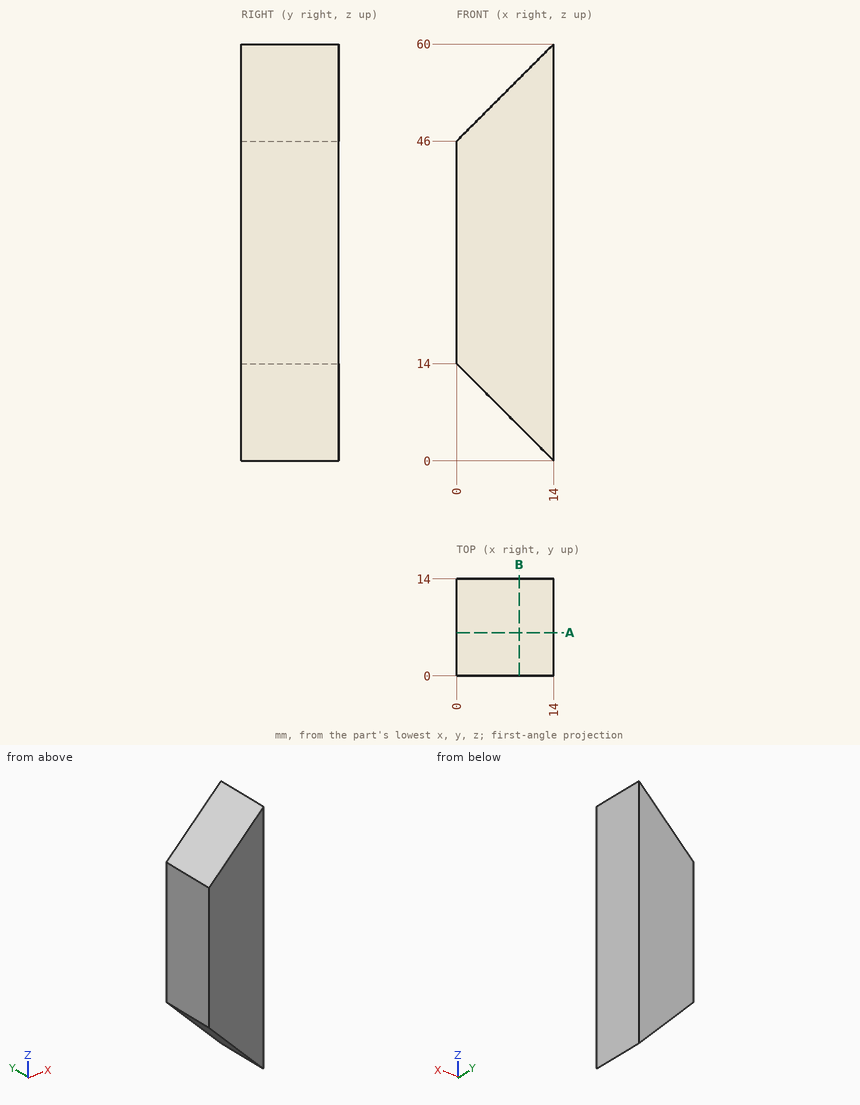
Check sheet for the drawn part. Datum: minimum x, y, z corner. Units: mm. Round coordinates to 2 decimals unless told otherwise and drop trailing zeros. Write each loop counter-clockwise with the first axis right and the second up, starting at its lowest first coordinate (ties: lowest second). Pieces come first, ordered by that corner, then holes. Notation, with made-up numbers: (64, 89.25) - (104, 89.25) arc R22 cw to (104, 111.25) - close; hole circle Ø10 at (-19, 16.5). An arc over 180 degrees is marked (long way). Write each question's results on one line, items separated by ' | '.
(1) Depth check by flat-ended pin: pin 1 Ø2 at (x, y) = (4, 2.5) entering from +Z; pin 2 Ø5 at (x, z) = (9, 31) entering from -Y. Enter the tip coordinate at first touch or a pass-through.
Computed:
pin 1: stops at z = 51 | pin 2: stops at y = 0
(2) Sectioned sample at B-B, the plane x = 9. Enter the section's corners in (y, z).
Computed:
outline: (0, 5) - (14, 5) - (14, 55) - (0, 55) - close
(3) Sectioned sample at A-A, the plane y = 6.25. Enter the section's corners in (x, z).
Computed:
outline: (0, 14) - (14, 0) - (14, 60) - (0, 46) - close
(4) Thickness scan on probe 1 along Z at (x, y) = (5.5, 5.75); probe 2 along Z at (x, y) = (9.5, 10.25); probe 3 along X at (y, z) = (3.25, 53.5). Record the ranges inside material, lowest first. Write a range as from..to.
Computed:
probe 1: z = 8.5..51.5 | probe 2: z = 4.5..55.5 | probe 3: x = 7.5..14
